The model under review builds one solid part; all positions refer to its coordinate system, in mm. A direction names the side the tool comes from. Give positions to 0.01 mm unless a question says otherwise; leave off trailing zeros. Write each loop counter-clockwise with the first axis right and the second up, starting at its lowest first coordinate (ties: lowest second). Pieces come first, ordered by that corner, then holes. Notation, with made-up numbers: (-31, 53) -> (-7, 53) arc R13 cw to (-7, 72) -> close; hole circle Ø8 at (-22.5, -33). An arc over 180 degrees is marked (long way). Use CSV: the item, a comma, the result in double quotes.
```python
from build123d import *

# Parameters (mm, degrees)
F1_DEPTH = 3
F3_DEPTH = 3
F4_R     = 3


with BuildPart() as f1:
    # F0 (on Top) → F1 (new body)
    with BuildSketch(Plane.XY):
        Polygon((-230, 0), (0, 0), (0, 318.5), (-280, 318.5), (-588.845279, 71.5), (-513.5, 0), (-270, 0), (-270, 110), (-195, 110), (-195, 150), (-75, 150), (-75, 30), (-195, 30), (-195, 70), (-230, 70), align=None)
    extrude(amount=F1_DEPTH)

    # F2 (on face) → F3 (join)
    with BuildSketch(Plane(origin=(0, 318.5, 0), x_dir=(-1, 0, 0), z_dir=(0, 1, 0))):
        Polygon((0, 75), (0, 3), (280, 3), (280, 70), (145, 75), align=None)
    extrude(amount=-F3_DEPTH)

    # F4
    f4_edges = [f1.edges().sort_by_distance(p)[0] for p in [
        (-140, 315.5, 3),
        (-140, 318.5, 0),
    ]]
    fillet(f4_edges, radius=F4_R)


solid = f1.part
```
Q1. Consider section D-D (x = -206). Write out the cut boundary in (y, z).
Derived:
outline,"(0, 0) -> (70, 0) -> (70, 3) -> (0, 3) -> close; (110, 0) -> (315.5, 0) arc R3 ccw to (318.5, 3) -> (318.5, 72.74) -> (315.5, 72.74) -> (315.5, 6) arc R3 cw to (312.5, 3) -> (110, 3) -> close"
Q2. Consider section A-A (x = -85.5). Write out the cut boundary in (y, z), then the cut area to 4 significant figures.
Derived:
outline,"(0, 0) -> (30, 0) -> (30, 3) -> (0, 3) -> close; (150, 0) -> (315.5, 0) arc R3 ccw to (318.5, 3) -> (318.5, 75) -> (315.5, 75) -> (315.5, 6) arc R3 cw to (312.5, 3) -> (150, 3) -> close"
area,"811.5 mm2"
Q3. To check wall thickness, follow probe 1 along Z at (x, y) = (-536, 83.5); probe 2 along Y at (x, z) = (-94.5, 13.5). State the ranges of each line that lie inside material, in increasing order.
Derived:
probe 1,"z = 0 to 3"
probe 2,"y = 315.5 to 318.5"
Q4. Insertion check: pin 1 (1.5 mm diameter, centred on x = -192, y = 192, fed in from +Z); pin 2 (3 mm diameter, centred on x = -385.5, y = 76.5, fed in from -Z); pin 3 (0.9 mm diameter, centred on x = -234, z = 1.5, fed in from -Y); pin 4 (0.9 mm diameter, centred on y = 75, z = 1.5, fed in from -X). Each pin has a flat end and moves straight along its axis. Give the tip position at first contact, or say it passes through.
Derived:
pin 1,"stops at z = 3"
pin 2,"stops at z = 0"
pin 3,"stops at y = 110"
pin 4,"stops at x = -585.03"
Q5. Machinability: for faces 1 (the flat face through (-138, 315.5, 41)), 2 (the flat face through (-432.3, 196.7, 1.5)), which of the approach directions +Z, -Z, +X, -X, +Y, -Y give a long, thin tool a straight path to every point of the face, cutting with its end or side? Answer none if there is none.
Derived:
face 1,"+Z, +X, -X, -Y"
face 2,"+Z, -Z, -X, +Y"
Q6. Consider section B-B (y = 143.5). Write out the cut boundary in (x, z).
Derived:
outline,"(-498.82, 0) -> (-195, 0) -> (-195, 3) -> (-498.82, 3) -> close; (-75, 0) -> (0, 0) -> (0, 3) -> (-75, 3) -> close"
Q7. Consider section C-C (z = 13.5). Write out the cut boundary in (x, y).
Derived:
outline,"(-280, 315.5) -> (0, 315.5) -> (0, 318.5) -> (-280, 318.5) -> close"
